Could you check a few things on this drawing? It's one solid part, dimensions in mm from its lowest x, y, z. Round coordinates to 2 decimals unless told otherwise and drop trailing zeros. Order: outer loops, then holes, each group sorted by start corner. A loop starts at its lowest first (then second) coordinate and runs counter-clockwise, first axis right, second up. Notation, with made-up numbers: (-27, 49.25) - (-18, 49.25) arc R26 cw to (-18, 85.25) - close; hole circle Ø11 at (15.5, 9.25). An arc over 180 degrees is marked (long way). Use one line per item in the form item = value.
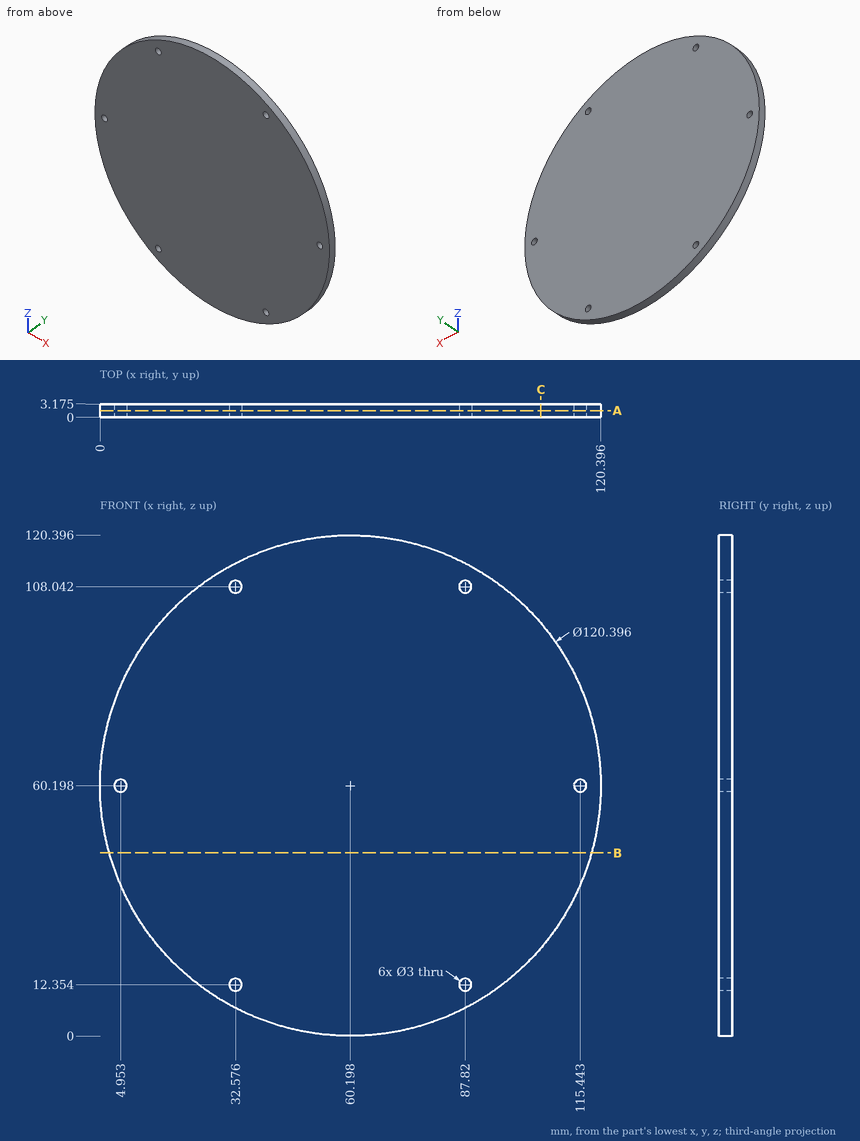
Item 1: I need wall thicknesses on L1, parallel to X at y = 1.65, z = 11 (1 decimal); L2, parallel to Z at x = 7.5, y = 2.6 (1 decimal); L3, parallel to X at y = 2.55, z = 82.5 (1 decimal). Which ranges of each line are inside material? Lowest first, please.
Found:
L1 = 25.5 to 31.9, 33.2 to 87.2, 88.5 to 94.9
L2 = 31.1 to 89.3
L3 = 4.3 to 116.1
Item 2: Imagine slicing it at A-A on y = 1.6. Please give me the cut outline in (x, z) (1 decimal).
Found:
outline = circle Ø120.4 at (60.2, 60.2); hole circle Ø3 at (5, 60.2); hole circle Ø3 at (32.6, 12.4); hole circle Ø3 at (32.6, 108); hole circle Ø3 at (87.8, 12.4); hole circle Ø3 at (87.8, 108); hole circle Ø3 at (115.4, 60.2)
Item 3: Imagine slicing it at B-B on z = 44. Please give me the cut outline in (x, y) (1 decimal).
Found:
outline = (2.2, 0) - (118.2, 0) - (118.2, 3.2) - (2.2, 3.2) - close
Item 4: Imagine slicing it at C-C on x = 106. Please give me the cut outline in (y, z) (1 decimal).
Found:
outline = (0, 21.1) - (3.2, 21.1) - (3.2, 99.3) - (0, 99.3) - close
